Source: CAD feature listing. Evaluate the final solid. Frame: model axes, mm. A direction names the side the tool comes from. Round coordinates to 2 decimals unless told otherwise and drop trailing zeros. Order: outer loops, then holes, each group sorted by start corner. A loop starts at its lowest first (then second) coordinate and runs counter-clockwise, first axis right, second up. Notation, with made-up numbers: (17.25, 81.25) -> (24.25, 81.25) arc R20 ccw to (24.25, 101.25) -> close; hole circle Ø5 at (45, 57). An arc over 180 degrees is marked (long way). One line per item, written item: value. Start each with the question number.
1) Reachability of faces 5 (the face through (-21, 8.5, 0)), 6 (the face through (0, 4, 0)), 7 (the face through (0, 0, 6)), 8 (the face through (-11.192, 7.226, 10.494)), 9 (the face through (0, 8.7, 0)) from +Z, -Z, +X, -X, +Y, -Y: full face, straight path, thin tool, end or side. Return the list, or none.
2) Pin query (flat end, axial travel): P1, Ø4, axis at x = -21, z = 5.5, coming from the +Y side; P2, Ø2, axis at x = 10, z = -10, coming from the +Y side; P3, Ø6, axis at x = 10, z = 1.5, coming from the -Y side; P4, Ø2.5, axis at x = 6, y = 6, coming from the +Z side. Return the tip coordinate at first contact, or that it passes through.
3) Section B-B (z = 0). Return the cut outline in (x, y), and give its area (3 significant figures).
4) Mould query, pull axis X, two halves, no side actions, for faces 1 (the face through (8.808, 7.226, 10.494)), 2 (the face through (-24.5, 5, 0)), 3 (the face through (-10.6, 7.23, -8.86)), 4 (the face through (21, 8.5, 0)). Classes: pulls with the +X half, pulls with the -X half, needs draft (parallel to the pull), parting line crosses it, or undercut.
5) Ray query, L1, parallel to Z at x = 10, y = 6.45; L2, parallel to X at y = 8.05, z = -10; L3, parallel to Z at x = 10, y = 6.35. Return the intervals inside material, ascending.
6) Section A-A (z = 7.25). Return the cut outline in (x, y).
```python
from build123d import *

# Parameters (mm, degrees)
EXTRUDE_1_DEPTH        = 49
SKETCH_2_W             = 34
SKETCH_2_H             = 4.7
EXTRUDE_2_DEPTH        = 0.1
SKETCH_3_W             = 34
SKETCH_3_H             = 4.6
EXTRUDE_3_DEPTH        = 0.1
SKETCH_4_W             = 34
SKETCH_4_H             = 27
EXTRUDE_4_DEPTH        = 0.5
CUT_EXTRUDE_1_DEPTH    = 34
SKETCH_6_W             = 9.8
SKETCH_6_H             = 0.3
CUT_EXTRUDE_2_DEPTH    = 45.558949718
DRAFT_1_ANGLE          = 45
DRAFT_2_ANGLE          = 45
DRAFT_3_ANGLE          = 45
HOLE_WIZARD_M2_1_D     = 2.58
HOLE_WIZARD_M2_1_DEPTH = 3.5
HOLE_WIZARD_M2_1_TIP   = 0.775110199
CHAMFER_1_SIZE         = 0.27
CHAMFER_2_SIZE         = 0.5
FILLET_1_R             = 0.3


with BuildPart() as part:
    # 草图1 → 凸台-拉伸1 (new body)
    with BuildSketch(Plane(origin=(-24.5, 0, 0), x_dir=(0, -1, 0), z_dir=(-1, 0, 0))):
        with BuildLine():
            Line((1, 13.4), (-8.5, 13.4))
            Line((-8.5, 13.4), (-8.5, -13.4))
            Line((-8.5, -13.4), (1, -13.4))
            Line((1, -13.4), (1, -6))
            Line((1, -6), (-0.408889, -6))
            ThreePointArc((-0.408889, -6), (-0.826571316, -5.367595703), (-1.51, -5.04))
            Line((-1.51, -5.04), (-1.51, -4.8))
            ThreePointArc((-1.51, -4.8), (-1.76, -4.55), (-2.01, -4.8))
            Line((-2.01, -4.8), (-2.01, -5.04))
            ThreePointArc((-2.01, -5.04), (-2.693428684, -5.367595703), (-3.111111, -6))
            Line((-3.111111, -6), (-4, -6))
            Line((-4, -6), (-4, 6))
            Line((-4, 6), (-3.111111, 6))
            ThreePointArc((-3.111111, 6), (-2.693428684, 5.367595703), (-2.01, 5.04))
            Line((-2.01, 5.04), (-2.01, 4.8))
            ThreePointArc((-2.01, 4.8), (-1.76, 4.55), (-1.51, 4.8))
            Line((-1.51, 4.8), (-1.51, 5.04))
            ThreePointArc((-1.51, 5.04), (-0.826571316, 5.367595703), (-0.408889, 6))
            Line((-0.408889, 6), (1, 6))
            Line((1, 6), (1, 13.4))
        make_face()
    extrude(amount=-EXTRUDE_1_DEPTH)

    # 草图2 → 凸台-拉伸2 (add)
    with BuildSketch(Plane(origin=(0, 0, -13.4), x_dir=(-1, 0, 0), z_dir=(0, 0, -1))):
        with Locations((0, 6.15)):
            Rectangle(SKETCH_2_W, SKETCH_2_H)
    extrude(amount=EXTRUDE_2_DEPTH)

    # 草图3 → 凸台-拉伸3 (add)
    with BuildSketch(Plane.XY.offset(13.4)):
        with Locations((0, 6.2)):
            Rectangle(SKETCH_3_W, SKETCH_3_H)
    extrude(amount=EXTRUDE_3_DEPTH)

    # 草图4 → 凸台-拉伸4 (add)
    with BuildSketch(Plane(origin=(0, 8.5, 0), x_dir=(-1, 0, 0), z_dir=(0, 1, 0))):
        Rectangle(SKETCH_4_W, SKETCH_4_H)
    extrude(amount=EXTRUDE_4_DEPTH)

    # 草图5 → 切除-拉伸1 (cut)
    with BuildSketch(Plane(origin=(17, 0, 0), x_dir=(0, 0, -1), z_dir=(1, 0, 0))):
        with BuildLine():
            Line((-13.5, 6.444948974), (-13.5, 5.955051026))
            ThreePointArc((-13.5, 5.955051026), (-13.4, 6.2), (-13.5, 6.444948974))
        make_face()
    extrude(amount=-CUT_EXTRUDE_1_DEPTH, mode=Mode.SUBTRACT)

    # 草图6 → 切除-拉伸2 (cut, through all)
    with BuildSketch(Plane(origin=(17, 0, 0), x_dir=(0, 0, -1), z_dir=(1, 0, 0))):
        with Locations((0, 8.85)):
            Rectangle(SKETCH_6_W, SKETCH_6_H)
    extrude(amount=-CUT_EXTRUDE_2_DEPTH, mode=Mode.SUBTRACT)

    # 拔模1
    draft_1_faces = [part.faces().sort_by_distance(p)[0] for p in [
        (0, 3.9, 13.45),
    ]]
    draft(draft_1_faces, Plane.XY.offset(13.5), DRAFT_1_ANGLE)

    # 拔模2
    draft_2_faces = [part.faces().sort_by_distance(p)[0] for p in [
        (0, 3.8, -13.45),
    ]]
    draft(draft_2_faces, Plane(origin=(24.5, 8.5, -13.4), x_dir=(-1, 0, 0), z_dir=(0, 0, -1)), DRAFT_2_ANGLE)

    # 拔模3
    draft_3_faces = [part.faces().sort_by_distance(p)[0] for p in [
        (0, 8.85, 4.9),
        (0, 8.85, -4.9),
    ]]
    draft(draft_3_faces, Plane(origin=(-24.5, 8.7, 4.9), x_dir=(0, 0, 1), z_dir=(0, 1, 0)), DRAFT_3_ANGLE)

    # M2 间隙孔1
    with Locations(Plane(origin=(0, 9, 0), x_dir=(1, 0, 0), z_dir=(0, 1, 0))):
        with Locations((10, -10), (-10, -10), (-10, 10), (10, 10)):
            Hole(HOLE_WIZARD_M2_1_D / 2, depth=HOLE_WIZARD_M2_1_DEPTH)
            with Locations((0, 0, -(HOLE_WIZARD_M2_1_DEPTH + HOLE_WIZARD_M2_1_TIP / 2))):  # 118° drill point
                Cone(0, HOLE_WIZARD_M2_1_D / 2, HOLE_WIZARD_M2_1_TIP, mode=Mode.SUBTRACT)

    # 倒角1
    chamfer_1_edges = [part.edges().sort_by_distance(p)[0] for p in [
        (0, -1, -13.4),
        (20.75, 8.5, -13.4),
        (20.75, 8.5, 13.4),
        (0, -1, 13.4),
        (-20.75, 8.5, -13.4),
        (-20.75, 8.5, 13.4),
    ]]
    chamfer(chamfer_1_edges, length=CHAMFER_1_SIZE)

    # 倒角2
    chamfer_2_edges = [part.edges().sort_by_distance(p)[0] for p in [
        (0, 9, 13.5),
        (0, 9, -13.5),
    ]]
    chamfer(chamfer_2_edges, length=CHAMFER_2_SIZE)

    # 圆角1
    fillet_1_edges = [part.edges().sort_by_distance(p)[0] for p in [
        (0, 0.408889, 6),
        (0, 1.51, 5.04),
        (0, 2.01, 5.04),
        (0, 3.111111, 6),
        (0, 4, 6),
        (0, 4, -6),
        (0, 3.111111, -6),
        (0, 2.01, -5.04),
        (0, 1.51, -5.04),
        (0, 0.408889, -6),
    ]]
    fillet(fillet_1_edges, radius=FILLET_1_R)


solid = part.part
```
Findings:
1. face 5: +Z, -Z, -X, +Y
1. face 6: +X, -X
1. face 7: +X, -X, -Y
1. face 8: +Y
1. face 9: +X, -X, +Y
2. P1: y = 8.5
2. P2: y = 5.33
2. P3: y = 4
2. P4: z = 13.5
3. outline: (-24.5, 4) -> (24.5, 4) -> (24.5, 8.5) -> (17, 8.5) -> (17, 8.7) -> (-17, 8.7) -> (-17, 8.5) -> (-24.5, 8.5) -> close
3. area: 227 mm2
4. face 1: undercut
4. face 2: pulls with the -X half
4. face 3: undercut
4. face 4: needs draft
5. L1: -13.5 to -11.29, -8.71 to 8.71, 11.29 to 13.5
5. L2: -24.5 to -11.29, -8.71 to 8.71, 11.29 to 24.5
5. L3: -13.5 to -11.29, -8.71 to 8.71, 11.29 to 13.43
6. outline: (-24.5, -1) -> (24.5, -1) -> (24.5, 8.5) -> (17, 8.5) -> (17, 9) -> (-17, 9) -> (-17, 8.5) -> (-24.5, 8.5) -> close
